Autodesk Inventor part; units mm, degrees
ref_plane "YZ Plane" through (0, 0, 0) normal (1, 0, 0) x (0, 1, 0)
ref_plane "XZ Plane" through (0, 0, 0) normal (0, 1, 0) x (-1, 0, 0)
ref_plane "XY Plane" through (0, 0, 0) normal (0, 0, 1) x (1, 0, 0)
sketch "Esboço1" plane through (0, 0, 0) normal (0, 0, 1) x (1, 0, 0)
  line L0 (-63.02, 0) -> (63.12, 0) construction
  line L1 (0, -42.02) -> (0, 42.12) construction
  line L2 (-45, 30) -> (45, 30)
  line L3 (45, 30) -> (45, -30)
  line L4 (45, -30) -> (-45, -30)
  line L5 (-45, -30) -> (-45, 30)
  line L6 (-15, 30) -> (45, 30) construction
  line L7 (45, 30) -> (45, 0) construction
  line L8 (45, 0) -> (-15, 0) construction
  line L9 (-15, 0) -> (-15, 30) construction
  line L10 (-15.1, 30.1) -> (45.1, 30.1)
  line L11 (45.1, 30.1) -> (45.1, -0.1)
  line L12 (45.1, -0.1) -> (-15.1, -0.1)
  line L13 (-15.1, -0.1) -> (-15.1, 30.1)
  line L14 (-25, 30) -> (-15, 30) construction
  line L15 (-15, 30) -> (-15, -30) construction
  line L16 (-15, -30) -> (-25, -30) construction
  line L17 (-25, -30) -> (-25, 30) construction
  line L18 (-45, 15) -> (45, 15) construction
  line L19 (-45, -15) -> (45, -15) construction
  line L20 (-20, -30) -> (-20, 30) construction
  line L21 (-35, 30) -> (-35, -30) construction
  line L22 (15, 30) -> (15, -30) construction
  circle A0 centre (-13, 2) radius 3
  point P0 (0, 0)
  point P1 (-20, 15)
  point P2 (-20, -15)
  point P3 (0, -15)
  point P4 (30, -15)
  point P5 (-35, 15)
  point P6 (-35, -15)
  point P7 (45, -0.1)
  point P8 (-15.1, 30)
  point P9 (-10.8576, -0.1)
  point P10 (-15.1, 4.1424)
  dimension "d0" = 60
  dimension "d1" = 90
  dimension "d2" = 60
  dimension "d3" = 30
  dimension "d4" = 0.1
  dimension "d5" = 10
  dimension "d6" = 30
  dimension "d7" = 30
  dimension "d17" = 6
  dimension "d18" = 2
  dimension "d19" = 2
extrude "Extrusão1" add sketch "Esboço1" against normal blind 10 contours L2 L13 A0 L12 L3 L4 L5 | L2 L3 L12 A0 L13 | A0 L12 L13 | L13 L12 A0
extrude "Extrusão2" cut sketch "Esboço1" against normal through all contours L2 L3 L12 A0 L13 | A0 L12 L13 | L13 L12 A0
hole "Furo1" at (0, -15, 0) at (30, -15, 0) at (-35, 15, 0) at (-35, -15, 0) direction (0, 0, -1) diameter 6.5 end through all countersink diameter 14.5 countersink angle 90
sketch "Esboço2" plane through (0, 0, -10) normal (0, 0, -1) x (-1, 0, 0)
  point P0 (0, 0)
  point P1 (20, 15)
  point P2 (20, -15)
hole "Furo2" at (-20, 15, -10) at (-20, -15, -10) direction (0, 0, 1) diameter 5.5 end through all countersink diameter 12.5 countersink angle 90
chamfer "Chanfro1" distance 1 angle 45 5 edges at (-45, 30, -5) (-15.1, 30, -5) (-45, -30, -5) (45, -30, -5) (45, -0.1, -5)
fillet "Arredondamento1" radius 2 2 edges at (-15.1, 4.1424, -5) (-10.8576, -0.1, -5)
equation "\"d18\" = 0.333333 * d17"
equation "\"d19\" = d18"
properties part number "Chapa Suporte 1L (Trilho Roletado)" material "Aluminio 1060"
The model under review builds one solid part; all positions refer to its coordinate system, in mm. A direction names the side the tool comes from. Round coordinates to 2 decimals unless told otherwise and drop trailing zeros. Write each loop counter-clockwise with the first axis right and the second up, starting at its lowest first coordinate (ties: lowest second). Pieces come first, ordered by that corner, then holes. Notation, with made-up numbers: (76, -30.75) - (102, -30.75) arc R14 cw to (102, -5.75) - close; hole circle Ø6 at (72, 40.5). An arc over 180 degrees is marked (long way). Answer as CSV lines item,"result". Start each with the question number.
(1) For faces 1 (the flat face through (-11, -6, -10)), 2 (the flat face through (-15.1, 17, -5)), list the 3-axis set-ups (+Z, -Z, +X, -X, +Y, -Y) from which the entire face can be reached by the end or side of a thin tool; tool diameter is ignored.
(2) To check wall thickness, follow line 1 (X direction, y = -15, z = -5.6); line 2 (Y direction, x = -35, z = -8.6); line 3 (X direction, y = -15, z = -8.6). State the ranges of each line that lie inside material, in increasing order.
(3) We need section A-A on x = 0. State the section outline as (y, z) points, plus the area to 3 significant figures.
(4) For pin 1 Ø10.5 at (x, y) = (-35, -15) entering from +Z; pin 2 Ø1 at (x, y) = (29, -18) entering from +Z; pin 3 Ø6 at (x, y) = (-35, 15) entering from +Z; pin 4 Ø8.5 at (x, y) = (0, -15) entering from +Z, all flat-tipped, find the tip position at first contact; note any pin that passes through.
(5) We need section D-D on y = -15. State the section outline as (x, z) points, plus the area to 3 significant figures.
(6) We need section C-C on x = -20. State the section outline as (y, z) points.
(7) Draft analysis for pull direction Y (two halves, no side actions). For faces 3 (the conical face through (-38.105, 13.385, -3.75)), 4 (the flat face through (-45, 0, -5)), 5 (the cylindrical face through (33.173, -14.295, -7.042)), 6 (the flat face through (1, -30, -5)), state which applies: pulls with the +Y half, pulls with the -Y half, needs draft (parallel to the pull), parting line crosses it, or undercut.
(8) We need section B-B on y = 15. State the section outline as (x, z) points.
Worked answers:
1,face 1,"-Z, +X, -X, +Y, -Y"
1,face 2,"+Z, -Z, +X, +Y"
2,line 1,"-45 to -38.25, -31.75 to -22.75, -17.25 to -3.25, 3.25 to 26.75, 33.25 to 45"
2,line 2,"-30 to -18.25, -11.75 to 11.75, 18.25 to 30"
2,line 3,"-45 to -38.25, -31.75 to -24.85, -15.15 to -3.25, 3.25 to 26.75, 33.25 to 45"
3,outline,"(-30, -10) - (-18.25, -10) - (-18.25, -4) - (-22.25, 0) - (-30, 0) - close; (-11.75, -10) - (-0.1, -10) - (-0.1, 0) - (-7.75, 0) - (-11.75, -4) - close"
3,area,"218 mm²"
4,pin 1,"z = -2"
4,pin 2,"z = -3.59"
4,pin 3,"through"
4,pin 4,"z = -3"
5,outline,"(-45, -10) - (-38.25, -10) - (-38.25, -4) - (-42.25, 0) - (-45, 0) - close; (-31.75, -10) - (-26.25, -10) - (-22.75, -6.5) - (-22.75, 0) - (-27.75, 0) - (-31.75, -4) - close; (-17.25, -6.5) - (-13.75, -10) - (-3.25, -10) - (-3.25, -4) - (-7.25, 0) - (-17.25, 0) - close; (3.25, -10) - (26.75, -10) - (26.75, -4) - (22.75, 0) - (7.25, 0) - (3.25, -4) - close; (33.25, -10) - (45, -10) - (45, 0) - (37.25, 0) - (33.25, -4) - close"
5,area,"590 mm²"
6,outline,"(-30, -10) - (-21.25, -10) - (-17.75, -6.5) - (-17.75, 0) - (-30, 0) - close; (-12.25, -6.5) - (-8.75, -10) - (8.75, -10) - (12.25, -6.5) - (12.25, 0) - (-12.25, 0) - close; (17.75, -6.5) - (21.25, -10) - (30, -10) - (30, 0) - (17.75, 0) - close"
7,face 3,"undercut"
7,face 4,"needs draft"
7,face 5,"undercut"
7,face 6,"pulls with the -Y half"
8,outline,"(-45, -10) - (-38.25, -10) - (-38.25, -4) - (-42.25, 0) - (-45, 0) - close; (-31.75, -10) - (-26.25, -10) - (-22.75, -6.5) - (-22.75, 0) - (-27.75, 0) - (-31.75, -4) - close; (-17.25, -6.5) - (-15.1, -8.65) - (-15.1, 0) - (-17.25, 0) - close"
